Here's how the part is built. I have some questions about the finished solid (model axes, mm). Round coordinates to 2 decimals unless told otherwise and drop trailing zeros. Order: outer loops, then holes, each group sorted by start corner. A loop starts at its lowest first (then second) coordinate and runs counter-clockwise, first axis right, second up.
Autodesk Inventor part; units mm, degrees
ref_plane "YZ Plane" through (0, 0, 0) normal (1, 0, 0) x (0, 1, 0)
ref_plane "XZ Plane" through (0, 0, 0) normal (0, 1, 0) x (-1, 0, 0)
ref_plane "XY Plane" through (0, 0, 0) normal (0, 0, 1) x (1, 0, 0)
sketch "Sketch3" plane through (0, 0, 0) normal (0, 1, 0) x (-1, 0, 0)
  line L0 (-17.78, -25.4) -> (17.78, -25.4)
  line L1 (17.78, -25.4) -> (17.78, 25.4)
  line L2 (17.78, 25.4) -> (-17.78, 25.4)
  line L3 (-17.78, 25.4) -> (-17.78, -25.4)
  line L4 (-17.78, -25.4) -> (17.78, 25.4) construction
  line L5 (17.78, -25.4) -> (-17.78, 25.4) construction
  point P0 (0, 0)
  dimension "d11" = 35.56
  dimension "d12" = 50.8
extrude "Extrusion3" add sketch "Sketch3" along normal blind 19.05
sketch "Sketch4" plane through (0, 19.05, 0) normal (0, 1, 0) x (1, 0, 0)
  circle A0 centre (0, 0) radius 15.875
  dimension "d15" = 31.75
extrude "Extrusion4" cut sketch "Sketch4" against normal blind 19.05
sketch "Sketch5" plane through (0, 19.05, 0) normal (0, 1, 0) x (1, 0, 0)
  line L0 (-17.6835, 25.5364) -> (55.9847, 25.5364) construction
  line L1 (-17.78, -25.4) -> (33.02, -25.4) construction
  circle A0 centre (12.2645, 19.8845) radius 1.778
  circle A1 centre (-12.2645, 19.8845) radius 1.778
  circle A2 centre (-12.2645, -19.8845) radius 1.778
  circle A3 centre (12.2645, -19.8845) radius 1.778
  point P0 (0, 0)
  point P1 (-17.78, 25.4)
  point P2 (17.78, -25.4)
  point P3 (17.78, 25.4)
  point P4 (0, 0)
  dimension "d20" = 3.556
  dimension "d21" = 3.556
  dimension "d22" = 3.556
  dimension "d23" = 3.556
extrude "Extrusion5" cut sketch "Sketch5" against normal blind 19.05
sketch "Sketch6" plane through (0, 19.05, 0) normal (0, 1, 0) x (1, 0, 0)
  line L0 (-17.78, -17.018) -> (17.78, -17.018)
  line L1 (-17.78, -17.018) -> (-17.78, -25.4)
  line L2 (-17.78, -25.4) -> (17.78, -25.4)
  line L3 (17.78, -25.4) -> (17.78, -17.018)
  point P0 (0, 0)
  point P1 (17.78, 25.4)
  point P2 (-17.78, 25.4)
  dimension "d26" = 42.418
extrude "Extrusion6" cut sketch "Sketch6" against normal blind 19.05
sketch "Sketch7" plane through (0, 19.05, 0) normal (0, 1, 0) x (1, 0, 0)
  circle A0 centre (-14.6899, -13.9279) radius 1.778
  circle A1 centre (14.6899, -13.9279) radius 1.778
  point P0 (0, 0)
  point P1 (-17.78, -17.018)
  dimension "d30" = 3.556
  dimension "d31" = 3.556
extrude "Extrusion7" cut sketch "Sketch7" against normal blind 19.05
properties part number "DPLX_P020_Camera Shroud Base_RevB"
1) If we section it at D-D (y = 14): Give the number of separate pieces and of enclosed holes in the cut face, plus the area to 3 significant figures.
2) If we section it at A-A (z = 0): Write out the boundary of the cut face in (x, y) (3 decimals).
3) If we section it at B-B (x = 0): Write out the boundary of the cut face in (y, z) (3 decimals).
4) We'd pull the mould along X, two halves only. Please class faces 1 (the flat face through (0, 9, -25.4)), 2 (the cylindrical face through (-3.441, 9.658, 15.497)), 3 (the flat face through (-17.78, 9, -4)): +X half, -X half, draft (parallel to the pull), parting line (faces both ways), or undercut.
5) I need wall thicknesses on line 1 (X direction, y = 7.75, z = 0.5); line 2 (X direction, y = 16.5, z = -20.5); line 3 (Z direction, x = -12.5, y = 8.5). Which ranges of each line are inside material? Lowest first, please.
6) If we section it at C-C (z = 13): Write out the boundary of the cut face in (x, y).
Solutions:
1. separate pieces: 1
1. enclosed holes: 5
1. area: 677 mm2
2. outline: (-17.78, 0) - (-15.875, 0) - (-15.875, 19.05) - (-17.78, 19.05) - close; (15.875, 0) - (17.78, 0) - (17.78, 19.05) - (15.875, 19.05) - close
3. outline: (0, -25.4) - (19.05, -25.4) - (19.05, -15.875) - (0, -15.875) - close; (0, 15.875) - (19.05, 15.875) - (19.05, 17.018) - (0, 17.018) - close
4. face 1: draft
4. face 2: undercut
4. face 3: -X half
5. line 1: x = -17.78 to -15.87, 15.87 to 17.78
5. line 2: x = -17.78 to -13.93, -10.6 to 10.6, 13.93 to 17.78
5. line 3: z = -25.4 to -21.65, -18.12 to -9.79, 9.79 to 17.02
6. outline: (-17.78, 0) - (-16.21, 0) - (-16.21, 19.05) - (-17.78, 19.05) - close; (-13.17, 0) - (-9.11, 0) - (-9.11, 19.05) - (-13.17, 19.05) - close; (9.11, 0) - (13.17, 0) - (13.17, 19.05) - (9.11, 19.05) - close; (16.21, 0) - (17.78, 0) - (17.78, 19.05) - (16.21, 19.05) - close
